from build123d import *

# Parameters (mm, degrees)
BOSS_EXTRUDE1_DEPTH = 12
SKETCH4_R           = 8
BOSS_EXTRUDE3_DEPTH = 66


# Read off the part's stored shape, not the designer's step: 5/8-11 Machine Threads Stud2
with BuildPart() as part:
    # Sketch1 → Boss-Extrude1 (new body)
    with BuildSketch(Plane.XY):
        Polygon((0, 0), (3.38231859, 18.162963808), (-10.656110181, 30.173619534), (-28.076857542, 24.021311453), (-31.459176132, 5.858347645), (-17.420747361, -6.152308082), align=None)
    extrude(amount=BOSS_EXTRUDE1_DEPTH)

    # Sketch4 → Boss-Extrude3 (add)
    with BuildSketch(Plane(origin=(0, 0, 0), x_dir=(-1, 0, 0), z_dir=(0, 0, -1))):
        with Locations((14.038428771, 12.010655726)):
            Circle(SKETCH4_R)
    extrude(amount=BOSS_EXTRUDE3_DEPTH)

    # 5/8-11 Machine Threads Stud2 outline → 5/8-11 Machine Threads Stud2 (revolve, cut)
    with BuildSketch(Plane(origin=(-14.038428771, 12.010655726, 0), x_dir=(1, 0, 0), z_dir=(0, -1, 0))):
        Polygon((6.56336, -66), (8, -66), (8, -41), (7.9375, -41), (7.9375, -64.62586), align=None)
    revolve(axis=Axis((-14.038428771, 12.010655726, 0), (0, 0, 1)), mode=Mode.SUBTRACT)


solid = part.part
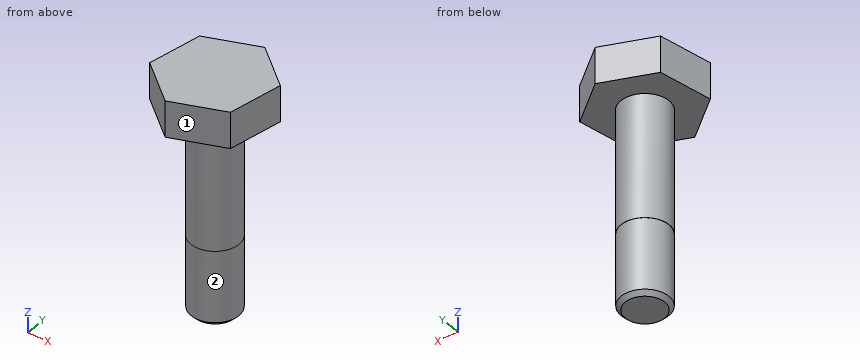
Verification items for the finished model (mm, model axes). Face numbers are marked on the shaded views. A direction names the side the tool comes from. Coordinates: 2 decimals unless noted, no trailing zeros. Order: outer loops, then holes, each group sorted by start corner. A loop starts at its lowest first (then second) coordinate and runs counter-clockwise, first axis right, second up.
Item 1: Section check D-D, the plane z = -18.5. Enter the section's corners in (x, y).
Filled in:
outline: circle Ø16 at (-14.04, 12.01)
Item 2: Section check C-C, the plane z = -56. Enter the section's corners in (x, y) (1 decimal).
Filled in:
outline: circle Ø15.9 at (-14, 12)
Item 3: Depth check by flat-ended pin: pin 1 (12 mm diameter, centred on x = -26.5, z = -50.5, fed in from +Y); pin 2 (1.5 mm diameter, centred on x = -25.5, y = 13.5, fed in from -Z); pin 3 (6 mm diameter, centred on x = -9.5, z = -16.5, fed in from +Y). Enter the tip coordinate at first touch or a pass-through.
Filled in:
pin 1: stops at y = 16.62
pin 2: stops at z = 0
pin 3: stops at y = 19.86
Item 4: Section check A-A, the plane z = 1. Enter the section's corners in (x, y), then the cut area to 3 significant figures.
Filled in:
outline: (-31.46, 5.86) - (-17.42, -6.15) - (0, 0) - (3.38, 18.16) - (-10.66, 30.17) - (-28.08, 24.02) - close
area: 887 mm2
Item 5: Access from +Z, -Z, +X, -X, +Y, -Y to the whole of each face (thin tool, end or side, straight path). Record for the marked faces 1 and 2.
Filled in:
face 1: +Z, -Z, +X, -Y
face 2: -Z
Item 6: Material ranges on L1, parallel to X at y = 12.5, z = -3.5; L2, parallel to Z at x = -2, y = 17.5; L3, parallel to X at y = 17.5, z = -29, recorded low to high.
Filled in:
L1: x = -22.02 to -6.05
L2: z = 0 to 12
L3: x = -19.86 to -8.22
Item 7: Section check B-B, the plane x = -4.5. Enter the section's corners in (y, z).
Filled in:
outline: (-1.59, 0) - (24.91, 0) - (24.91, 12) - (-1.59, 12) - close
